from build123d import *

# Parameters (mm, degrees)
F1_DEPTH      = 38.1
F3_DEPTH      = 35.56
F3_DEPTH_BACK = 42.926


with BuildPart() as f1:
    # F0 (on Front) → F1 (new body)
    with BuildSketch(Plane.XZ):
        Polygon((-67.434916, 27.502788), (-67.434916, -35.997212), (59.565084, -35.997212), (59.565084, 27.502788), (34.165084, 27.502788), (34.165084, -16.947212), (-42.034916, -16.947212), (-42.034916, 27.502788), align=None)
    extrude(amount=F1_DEPTH)

    # F2 (on Right) → F3 (join, two sides)
    with BuildSketch(Plane.YZ) as f3_sk:
        Polygon((0, 18.508689), (-39.34918, -16.759835), (0, -16.759835), align=None)
    extrude(amount=F3_DEPTH)
    extrude(f3_sk.sketch, amount=-F3_DEPTH_BACK)


solid = f1.part
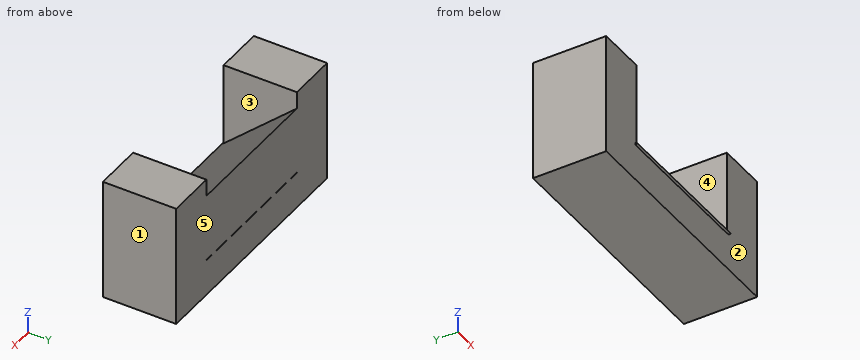
Could you check a few things on this model? Use its own coordinates, in mm. Face numbers are marked on the shaded views. A direction names the side the tool comes from. Round coordinates to 2 decimals unless told otherwise and drop trailing zeros. Loops run counter-clockwise (first coordinate to the right, second up) from the corner with the lowest first, then second, coordinate; pieces in that order, holes last. Notation, with made-up numbers: (-27.75, 69.25) -> (-20.75, 69.25) arc R22 ccw to (-20.75, 83.25) -> close; hole circle Ø3 at (47, 74). An arc over 180 degrees is marked (long way). Use CSV: the item, a comma, the result in double quotes.
(1) For the marked faces 4 and 5, which set-ups out of +Z, -Z, +X, -X, +Y, -Y let a thin tool reach every point of the face, with its end or its side?
Return value:
face 4,"+Z, -Y"
face 5,"+Z, -Z, +X, -X, +Y"
(2) Suppose I cut it at C-C on z = -6.5. Write out the boundary of the cut face in (x, y), plus the area to 3 significant figures.
Return value:
outline,"(-67.43, -38.1) -> (-42.03, -38.1) -> (-42.03, -27.9) -> (34.17, -27.9) -> (34.17, -38.1) -> (59.57, -38.1) -> (59.57, 0) -> (-67.43, 0) -> close"
area,"4,060 mm²"
(3) If we mould it in two halves opening along X, with no side actions, what happens to the marked faces 1, 2 and 3? For each: +X half, -X half, draft (parallel to the pull), parting line (faces both ways), or undercut.
Return value:
face 1,"+X half"
face 2,"draft"
face 3,"undercut"
(4) Suppose I cut it at B-B on y = -17. Write out the boundary of the cut face in (x, z), plus the area to 3 significant figures.
Return value:
outline,"(-67.43, -36) -> (59.57, -36) -> (59.57, 27.5) -> (34.17, 27.5) -> (34.17, 3.27) -> (-42.03, 3.27) -> (-42.03, 27.5) -> (-67.43, 27.5) -> close; hole (-42.03, -16.95) -> (34.17, -16.95) -> (34.17, -16.76) -> (-42.03, -16.76) -> close"
area,"6,200 mm²"
(5) Will these pins go through, and if not, where does the flat tip stop? pin 1 Ø10 at (x, z) = (31.5, 5) entering from +Y; pin 2 Ø2 at (x, z) = (-32, -18) entering from -Y; pin 3 Ø0.6 at (y, z) = (-38.5, -16) entering from +X; pin 4 Ø19 at (x, z) = (-30, 11) entering from -Y.
Return value:
pin 1,"stops at y = 0"
pin 2,"stops at y = -38.1"
pin 3,"stops at x = 35.56"
pin 4,"stops at y = -18.98"
(6) Suppose I cut it at D-D on x = 42. Write out the boundary of the cut face in (y, z).
Return value:
outline,"(-38.1, -36) -> (0, -36) -> (0, 27.5) -> (-38.1, 27.5) -> close"
(7) Suppose I cut it at A-A on x = -26. Write out the boundary of the cut face in (y, z), plus the area to 3 significant figures.
Return value:
outline,"(-39.35, -16.76) -> (0, -16.76) -> (0, 18.51) -> close; (-38.1, -36) -> (0, -36) -> (0, -16.95) -> (-38.1, -16.95) -> close"
area,"1,420 mm²"
(8) If I drill on probe 1 along X at (y, z) = (-32, 15.5); probe 2 along Y at (x, z) = (-0.5, -24.5); probe 3 along Z at (x, y) = (16, -32), over which ranges is the centre line in solid material (lowest first)? Write a range as [from, to].
Return value:
probe 1,"x = [-67.43, -42.03], [34.17, 59.57]"
probe 2,"y = [-38.1, 0]"
probe 3,"z = [-36, -16.95], [-16.76, -10.17]"
